```python
from build123d import *

# Parameters (mm, degrees)
CROQUIS1_W              = 50
CROQUIS1_H              = 100
CROQUIS1_W_2            = 45
CROQUIS1_H_2            = 95
SALIENTE_EXTRUIR1_DEPTH = 800
CROQUIS2_W              = 1600
CROQUIS2_H              = 30
CORTAR_EXTRUIR1_DEPTH   = 5
CROQUIS8_R              = 7.14375
CORTAR_EXTRUIR2_DEPTH   = 130


with BuildPart() as part:
    # Croquis1 → Saliente-Extruir1 (new, symmetric)
    with BuildSketch(Plane.XY):
        Rectangle(CROQUIS1_W, CROQUIS1_H)
        Rectangle(CROQUIS1_W_2, CROQUIS1_H_2, mode=Mode.SUBTRACT)
    extrude(amount=SALIENTE_EXTRUIR1_DEPTH, both=True)

    # Croquis2 → Cortar-Extruir1 (cut)
    with BuildSketch(Plane(origin=(25, 0, 0), x_dir=(0, 0, -1), z_dir=(1, 0, 0))):
        Rectangle(CROQUIS2_W, CROQUIS2_H)
    extrude(amount=-CORTAR_EXTRUIR1_DEPTH, mode=Mode.SUBTRACT)

    # Croquis8 → Cortar-Extruir2 (cut)
    with BuildSketch(Plane(origin=(25, 50, 0), x_dir=(0, 0, 1), z_dir=(0, -1, 0))):
        with Locations(Location((0, 25, 0), (0, 0, 180))):
            Circle(CROQUIS8_R)
        with Locations(Location((100, 25, 0), (0, 0, 180))):
            Circle(CROQUIS8_R)
        with Locations(Location((200, 25, 0), (0, 0, 180))):
            Circle(CROQUIS8_R)
        with Locations(Location((300, 25, 0), (0, 0, 180))):
            Circle(CROQUIS8_R)
        with Locations(Location((400, 25, 0), (0, 0, 180))):
            Circle(CROQUIS8_R)
        with Locations(Location((500, 25, 0), (0, 0, 180))):
            Circle(CROQUIS8_R)
        with Locations(Location((600, 25, 0), (0, 0, 180))):
            Circle(CROQUIS8_R)
        with Locations(Location((700, 25, 0), (0, 0, 180))):
            Circle(CROQUIS8_R)
        with Locations(Location((-100, 25, 0), (0, 0, 180))):
            Circle(CROQUIS8_R)
        with Locations(Location((-200, 25, 0), (0, 0, 180))):
            Circle(CROQUIS8_R)
        with Locations(Location((-300, 25, 0), (0, 0, 180))):
            Circle(CROQUIS8_R)
        with Locations(Location((-400, 25, 0), (0, 0, 180))):
            Circle(CROQUIS8_R)
        with Locations(Location((-500, 25, 0), (0, 0, 180))):
            Circle(CROQUIS8_R)
        with Locations(Location((-600, 25, 0), (0, 0, 180))):
            Circle(CROQUIS8_R)
        with Locations(Location((-700, 25, 0), (0, 0, 180))):
            Circle(CROQUIS8_R)
    extrude(amount=CORTAR_EXTRUIR2_DEPTH, mode=Mode.SUBTRACT)


solid = part.part
```
Input: part model. Units: mm. Frame: model coordinates. A direction names the side the tool comes from. Coordinates: 2 decimals unless noted, no trailing zeros. Write each loop counter-clockwise with the first axis right and the second up, starting at its lowest first coordinate (ties: lowest second). Pieces come first, ordered by that corner, then holes.
1) Set-up query: faces 5 (the flat face through (-22.5, -1, 11)), 6 (the flat face through (-24, 0, -800)). Return all of +Z, -Z, +X, -X, +Y, -Y with unobstructed straight access to the full face (end or side cutting, diameter ignored); none if empty.
2) Material intervals for line 1 along X through (y, z) = (48.5, -600); line 2 along Y through (x, z) = (20.5, -306); line 3 along X through (y, z) = (15.5, 36.5), sorted ascending.
3) Mould query, pull axis X, two halves, no side actions, for faces 1 (the flat face through (0, -47.5, 11)), 2 (the flat face through (0, 47.5, 11)), 3 (the flat face through (0, -50, 11)), 4 (the flat face through (25, 32, 11)). Classes: pulls with the +X half, pulls with the -X half, needs draft (parallel to the pull), parting line crosses it, or undercut.
4) Section B-B on z = 271.5. Output: boundary loops of the cut face in (x, y).
5) Section A-A on y = 28.5. Output: boundary loops of the cut face in (x, z).
6) Pin query (flat end, axial travel): pin 1 Ø8.5 at (x, z) = (0, -700) entering from -Y; pin 2 Ø1 at (y, z) = (13, 185.5) entering from +X. Return the tip coordinate at first contact, or that it passes through.
Check result:
1. face 5: +Z, -Z
1. face 6: -Z, +X, -X, +Y, -Y
2. line 1: x = -25 to -7.14, 7.14 to 25
2. line 2: y = -50 to -47.5, 47.5 to 50
2. line 3: x = -25 to -22.5, 22.5 to 25
3. face 1: undercut
3. face 2: undercut
3. face 3: needs draft
3. face 4: pulls with the +X half
4. outline: (-25, -50) - (25, -50) - (25, -15) - (22.5, -15) - (22.5, -47.5) - (-22.5, -47.5) - (-22.5, 47.5) - (22.5, 47.5) - (22.5, 15) - (25, 15) - (25, 50) - (-25, 50) - close
5. outline: (-25, -800) - (-22.5, -800) - (-22.5, 800) - (-25, 800) - close; (22.5, -800) - (25, -800) - (25, 800) - (22.5, 800) - close
6. pin 1: passes through
6. pin 2: stops at x = -22.5
